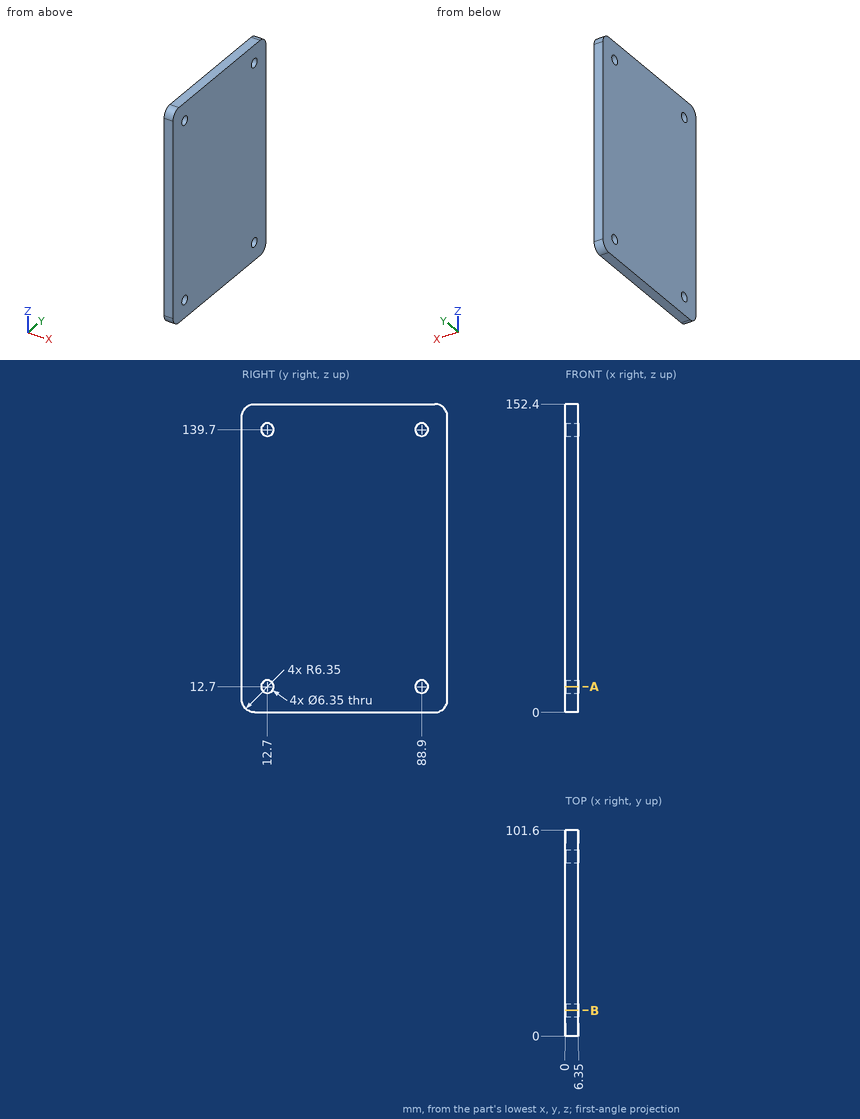
Study the drawing (mm; zero at the part's minimum x, y, z) and answer. Give positions to 0.01 mm unless a question says otherwise; leave off trailing zeros. Loops run counter-clockwise (first coordinate to the right, second up) from the corner with the lowest first, then second, coordinate; pieces in that order, holes last. Notation, with made-up numbers: (-11.75, 10) - (30.25, 10) arc R11 ccw to (30.25, 18) - close; hole circle Ø8 at (27, 48.25). An arc over 180 degrees is marked (long way). Return JSON: item names as keys, results as strings. Group by question number.
1. Find section B-B (y = 12.7). Write down the section's boundary in (x, z) (3 decimals), then the cut area to 3 significant figures.
2. Find section A-A (z = 12.7). Write down the section's boundary in (x, y) (3 decimals).
3. Straight lines are drawn through the part: line 1 (Y direction, x = 2, z = 139.7) (3 decimals); line 2 (Y direction, x = 1.5, z = 138); line 3 (Z direction, x = 3.5, y = 86). For each, find the intervals that lie inside material, in ascending order. Write a range as [from, to].
Verdict:
{
 "1": {"outline": "(0, 0) - (6.35, 0) - (6.35, 9.525) - (0, 9.525) - close; (0, 15.875) - (6.35, 15.875) - (6.35, 136.525) - (0, 136.525) - close; (0, 142.875) - (6.35, 142.875) - (6.35, 152.4) - (0, 152.4) - close", "area": "887 mm^2"},
 "2": {"outline": "(0, 0) - (6.35, 0) - (6.35, 9.525) - (0, 9.525) - close; (0, 15.875) - (6.35, 15.875) - (6.35, 85.725) - (0, 85.725) - close; (0, 92.075) - (6.35, 92.075) - (6.35, 101.6) - (0, 101.6) - close"},
 "3": {"line 1": "y = [0, 9.525], [15.875, 85.725], [92.075, 101.6]", "line 2": "y = [0, 10.02], [15.38, 86.22], [91.58, 101.6]", "line 3": "z = [0, 11.41], [13.99, 138.41], [140.99, 152.4]"}
}
